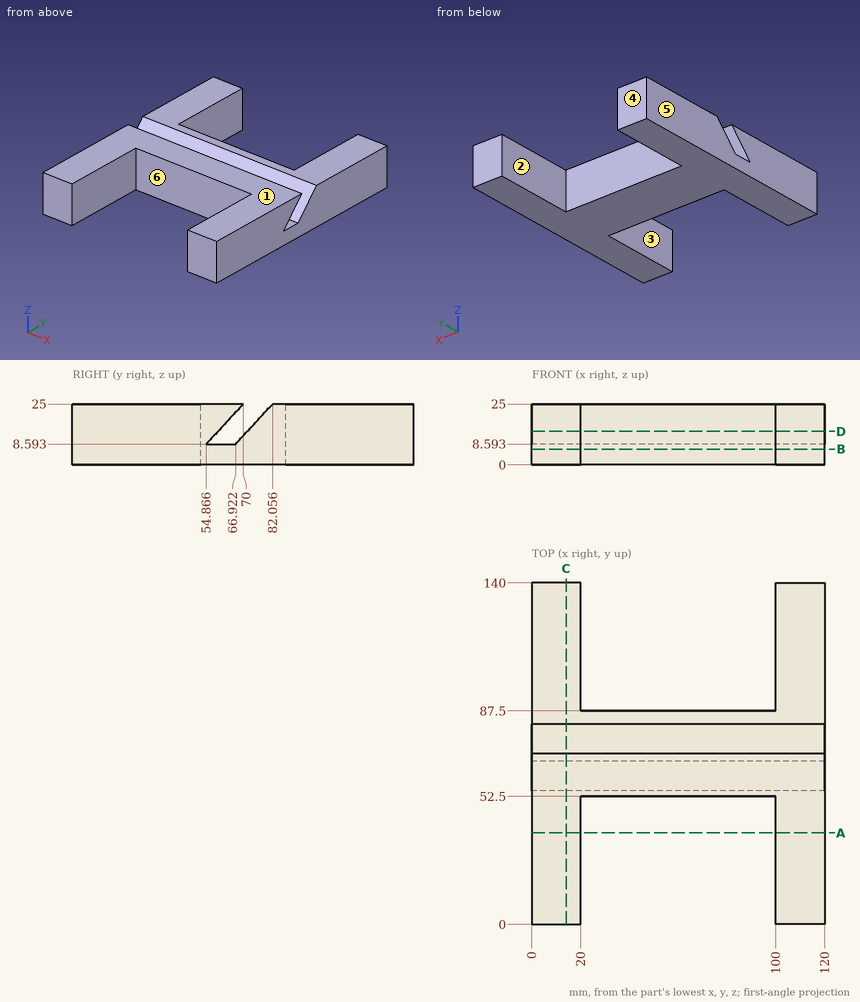
Could you check a few things on this drawing? It's one solid part, dimensions in mm from its lowest x, y, z. A direction names the side the tool comes from. Round coordinates to 2 decimals unless told otherwise and drop trailing zeros. Loops run counter-clockwise (first coordinate to the right, second up) from the corner with the lowest first, then second, coordinate; pieces in that order, holes last.
Q1. I want a section at A-A (y = 37.5). Write out the boundary of the cut face in (x, z).
Q2. Please list where these lines run through material, in increasing order: L1, parallel to X at y = 99.5, z = 9.25; L2, parallel to Y at x = 80, z = 6; L3, parallel to Y at x = 72.5, z = 19 (1 decimal).
Q3. On a 3-axis mill with a long thin cutter (end or side, diameter ignored), from which of +Z, -Z, +X, -X, +Y, -Y can I reach the whole of each face in a straight line? I mean the marked faces 1, 2 and 3. Say none if no direction works.
Q4. I want a section at D-D (z = 13.75). Write out the boundary of the cut face in (x, y), and give its area (3 significant figures).
Q5. For P1, Ø6, axis at x = 64, z = 2.5, coming from the +Y side; P2, Ø5, axis at x = 17.5, y = 77.5, coming from the +Z side, each with a flat end and sliding along its axis, tell me the tip position at first contact or that it passes through.
Q6. Thinking about a two-plate mould opening in X: for the marked faces 4, 5 and 6, which applies, pulls with the +X half, pulls with the -X half, needs draft (parallel to the pull), parting line crosses it, or undercut?
Q7. I want a section at C-C (x = 14). Write out the boundary of the cut face in (y, z) (1 decimal), and give its area (3 significant figures).
Q8. I want a section at B-B (z = 6.5). Write out the boundary of the cut face in (x, y), and give its area (3 significant figures).
Answer below:
1. outline: (0, 0) - (20, 0) - (20, 25) - (0, 25) - close; (100, 0) - (120, 0) - (120, 25) - (100, 25) - close
2. L1: x = 0 to 20, 100 to 120
2. L2: y = 52.5 to 87.5
2. L3: y = 52.5 to 64.5, 76.5 to 87.5
3. face 1: +Z, +X, -X, +Y, -Y
3. face 2: +Z, -Z, +Y
3. face 3: +Z, -Z, -Y
4. outline: (0, 0) - (20, 0) - (20, 52.5) - (100, 52.5) - (100, 0) - (120, 0) - (120, 59.62) - (0, 59.62) - close; (0, 71.68) - (120, 71.68) - (120, 140) - (100, 140) - (100, 87.5) - (20, 87.5) - (20, 140) - (0, 140) - close
4. area: 6,950 mm2
5. P1: stops at y = 87.5
5. P2: stops at z = 22.77
6. face 4: needs draft
6. face 5: pulls with the -X half
6. face 6: undercut
7. outline: (0, 0) - (140, 0) - (140, 25) - (82.1, 25) - (66.9, 8.6) - (54.9, 8.6) - (70, 25) - (0, 25) - close
7. area: 3,300 mm2
8. outline: (0, 0) - (20, 0) - (20, 52.5) - (100, 52.5) - (100, 0) - (120, 0) - (120, 140) - (100, 140) - (100, 87.5) - (20, 87.5) - (20, 140) - (0, 140) - close
8. area: 8,400 mm2
